```python
from build123d import *

# Parameters (mm, degrees)
F0_W      = 1060.45
F0_H      = 2101.85
F1_DEPTH  = 101.6
F2_W      = 19.05
F2_H      = 50.8
F3_DEPTH  = 2101.85
F4_W      = 41.91
F4_H      = 139.7
F5_DEPTH  = 3.175
F6_R      = 3.175
F10_W     = 38.1
F10_H     = 12.7
F11_DEPTH = 15.87246
F12_R     = 19.05
F13_DEPTH = 6.35
F15_DEPTH = 25.4


with BuildPart() as f1:
    # F0 (on Front) → F1 (new body)
    with BuildSketch(Plane.XZ):
        Rectangle(F0_W, F0_H)
    extrude(amount=F1_DEPTH)

    # F2 (on face) → F3 (cut, through all)
    with BuildSketch(Plane.XY.offset(1050.925)):
        with Locations((-520.7, -76.2)):
            Rectangle(F2_W, F2_H)
    extrude(amount=-F3_DEPTH, mode=Mode.SUBTRACT)

    # F4 (on face) → F5 (cut)
    with BuildSketch(Plane.YZ.offset(530.225)):
        with Locations((-20.955, -796.925)):
            Rectangle(F4_W, F4_H)
        with Locations((-20.955, -250.825)):
            Rectangle(F4_W, F4_H)
        with Locations((-20.955, 295.275)):
            Rectangle(F4_W, F4_H)
        with Locations((-20.955, 841.375)):
            Rectangle(F4_W, F4_H)
    extrude(amount=-F5_DEPTH, mode=Mode.SUBTRACT)

    # F9: sweep along a path in F8
    with BuildLine(Plane(origin=(-434.975, 0, 0), x_dir=(0, -1, 0), z_dir=(-1, 0, 0))) as f9_path:
        Line((101.6, -111.125), (120.65, -111.125))
        ThreePointArc((120.65, -111.125), (125.1401280605, -112.9848719395), (127, -117.475))
        Line((127, -117.475), (127, -155.575))
        ThreePointArc((127, -155.575), (125.1401280605, -160.0651280606), (120.65, -161.925))
        Line((120.65, -161.925), (101.6, -161.925))
    # F6 (on face) → F9 (sweep)
    with BuildSketch(Plane.XZ.offset(101.6)):
        with Locations((-434.975, -111.125)):
            Circle(F6_R)
    sweep(path=f9_path.line)

    # F10 (on face) → F11 (join)
    with BuildSketch(Plane(origin=(0, 0, 0), x_dir=(-1, 0, 0), z_dir=(0, 1, 0))):
        with Locations((460.375, 1043.78125)):
            Rectangle(F10_W, F10_H)
    extrude(amount=F11_DEPTH)

    # F12 (on face) → F13 (join)
    with BuildSketch(Plane.XZ.offset(101.6)):
        with Locations((-434.975, -34.925)):
            Circle(F12_R)
    extrude(amount=F13_DEPTH)

    # F14 (on face) → F15 (cut)
    with BuildSketch(Plane.XZ.offset(107.95)):
        with BuildLine():
            Line((-438.4902051281, -47.4607607431), (-438.4902051281, -53.6478692488))
            ThreePointArc((-438.4902051281, -53.6478692488), (-434.975, -53.975), (-431.4597948719, -53.6478692488))
            Line((-431.4597948719, -53.6478692488), (-431.4597948719, -47.4607607431))
            Line((-431.4597948719, -47.4607607431), (-433.7515848637, -47.4607607431))
            Line((-433.7515848637, -47.4607607431), (-433.7515848637, -44.9119880795))
            Line((-433.7515848637, -44.9119880795), (-431.7125695705, -42.7710190415))
            Line((-431.7125695705, -42.7710190415), (-433.9554923534, -41.9554114342))
            Line((-433.9554923534, -41.9554114342), (-431.9164770603, -40.2222499251))
            Line((-431.9164770603, -40.2222499251), (-431.9164770603, -35.634458065))
            Line((-431.9164770603, -35.634458065), (-433.5476773739, -33.5954427719))
            Line((-433.5476773739, -33.5954427719), (-433.5476773739, -31.2505699694))
            Line((-433.5476773739, -31.2505699694), (-431.9164770603, -31.2505699694))
            Line((-431.9164770603, -31.2505699694), (-431.9164770603, -28.5998471081))
            Line((-431.9164770603, -28.5998471081), (-434.975, -26.0510761291))
            Line((-434.975, -26.0510761291), (-438.0335229397, -28.5998471081))
            Line((-438.0335229397, -28.5998471081), (-438.0335229397, -31.2505699694))
            Line((-438.0335229397, -31.2505699694), (-436.4023226261, -31.2505699694))
            Line((-436.4023226261, -31.2505699694), (-436.4023226261, -33.5954427719))
            Line((-436.4023226261, -33.5954427719), (-438.0335229397, -35.634458065))
            Line((-438.0335229397, -35.634458065), (-438.0335229397, -40.2222499251))
            Line((-438.0335229397, -40.2222499251), (-435.9945076466, -41.9554114342))
            Line((-435.9945076466, -41.9554114342), (-438.2374304295, -42.7710190415))
            Line((-438.2374304295, -42.7710190415), (-436.1984151363, -44.9119880795))
            Line((-436.1984151363, -44.9119880795), (-436.1984151363, -47.4607607431))
            Line((-436.1984151363, -47.4607607431), (-438.4902051281, -47.4607607431))
        make_face()
    extrude(amount=-F15_DEPTH, mode=Mode.SUBTRACT)


solid = f1.part
```
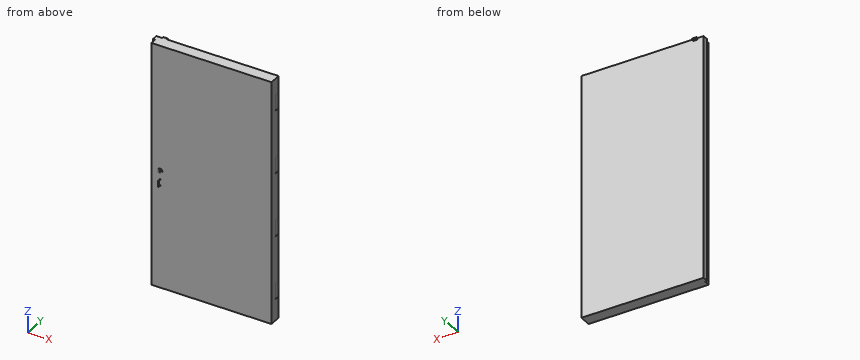
For this review, take the finished solid that the model builds, in its own axes (mm). Coordinates: 2 decimals unless noted, no trailing zeros. Write each loop counter-clockwise with the first axis right and the second up, starting at its lowest first coordinate (ties: lowest second). Pieces come first, ordered by that corner, then holes.
(1) Add section A-A on z = 831. Give the boundary of the cut face in (x, y) (3 decimals).
(2) Add section C-C on z = 195. Give the boundary of the cut face in (x, y) (3 decimals), then the cut area to 3 significant figures.
(3) Add section B-B on x = -31.5. Give the boundary of the cut face in (y, z) (3 decimals).
(4) Wall thickness on probe 1 along Y at (x, z) = (-24.5, 380.5); probe 2 along X at (y, z) = (-12, 775) (3 decimals); probe 3 along X at (y, z) = (-89.5, 824.5) (3 decimals): over which ranges is each line inside the solid? List them lowest first.
(5) For pin 1 Ø2.5 at (x, z) = (528, -275) entering from +Y; pin 2 Ø10 at (y, z) = (8, 1041) entering from -X (3 decimals); pin 3 Ø1 at (y, z) = (-66.5, -93.5) entering from -X (3 decimals), all flat-tipped, find the tip position at first contact; note any pin that passes through.
Answer sheet:
1. outline: (-530.225, -50.8) - (-511.175, -50.8) - (-511.175, -101.6) - (530.225, -101.6) - (530.225, -41.91) - (527.05, -41.91) - (527.05, 0) - (-530.225, 0) - close
2. outline: (-530.225, -50.8) - (-511.175, -50.8) - (-511.175, -101.6) - (530.225, -101.6) - (530.225, 0) - (-530.225, 0) - close
2. area: 107,000 mm2
3. outline: (-101.6, -1050.925) - (0, -1050.925) - (0, 1050.925) - (-101.6, 1050.925) - close
4. probe 1: y = -101.6 to 0
4. probe 2: x = -530.225 to 527.05
4. probe 3: x = -511.175 to 530.225
5. pin 1: stops at y = 0
5. pin 2: stops at x = -479.425
5. pin 3: stops at x = -511.175
